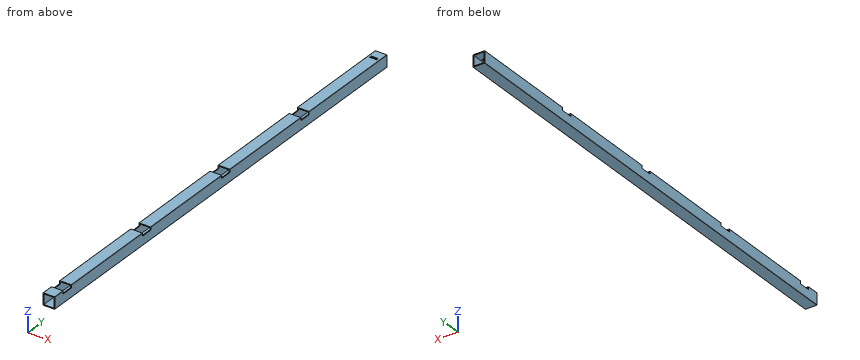
from build123d import *

# Parameters (mm, degrees)
SKETCH1_W           = 17
SKETCH1_H           = 17
BOSS_EXTRUDE1_DEPTH = 796.5
SKETCH3_W           = 12
SKETCH3_H           = 4
CUT_EXTRUDE1_DEPTH  = 10
SKETCH5_W           = 5
SKETCH5_H           = 20
CUT_EXTRUDE2_DEPTH  = 798.002038893


with BuildPart() as part:
    # Sketch1 → Boss-Extrude1 (new body)
    with BuildSketch(Plane(origin=(0, 0, 0), x_dir=(1, 0, 0), z_dir=(0, 1, 0))):
        with BuildLine():
            Line((0.5, 0), (19.5, 0))
            ThreePointArc((19.5, 0), (19.853553391, 0.146446609), (20, 0.5))
            Line((20, 0.5), (20, 19.5))
            ThreePointArc((20, 19.5), (19.853553391, 19.853553391), (19.5, 20))
            Line((19.5, 20), (0.5, 20))
            ThreePointArc((0.5, 20), (0.146446609, 19.853553391), (0, 19.5))
            Line((0, 19.5), (0, 0.5))
            ThreePointArc((0, 0.5), (0.146446609, 0.146446609), (0.5, 0))
        make_face()
        with Locations((10, 10)):
            Rectangle(SKETCH1_W, SKETCH1_H, mode=Mode.SUBTRACT)
    extrude(amount=BOSS_EXTRUDE1_DEPTH)

    # Sketch3 → Cut-Extrude1 (cut)
    with BuildSketch(Plane.XY):
        with Locations((10, 779.5)):
            Rectangle(SKETCH3_W, SKETCH3_H)
    extrude(amount=-CUT_EXTRUDE1_DEPTH, mode=Mode.SUBTRACT)

    # Sketch5 → Cut-Extrude2 (cut, through all)
    with BuildSketch(Plane.ZY):
        with Locations((-2.5, 600)):
            Rectangle(SKETCH5_W, SKETCH5_H)
        with Locations((-2.5, 410)):
            Rectangle(SKETCH5_W, SKETCH5_H)
        with Locations((-2.5, 220)):
            Rectangle(SKETCH5_W, SKETCH5_H)
        with Locations((-2.5, 30)):
            Rectangle(SKETCH5_W, SKETCH5_H)
    extrude(amount=-CUT_EXTRUDE2_DEPTH, mode=Mode.SUBTRACT)


solid = part.part
Design review of the part built by this model. Coordinates are the model's own, in mm. Round coordinates to 2 decimals unless told otherwise and drop trailing zeros. Write each loop counter-clockwise with the first axis right and the second up, starting at its lowest first coordinate (ties: lowest second). Pieces come first, ordered by that corner, then holes. Notation, with made-up numbers: (28.5, -6) - (80.5, -6) arc R24 ccw to (80.5, 24) - close; hole circle Ø6 at (56.5, 23.5). An arc over 180 degrees is marked (long way). Return JSON: item names as keys, results as strings. Group by question number.
Item 1: We need section B-B on z = -13.25. Write out the cut boundary in (x, y).
Item 2: Insertion check: P1, Ø0.8, axis at x = 19.5, y = 600, coming from the +Z side; P2, Ø6, axis at x = 7.5, z = -13, coming from the +Y side; P3, Ø5.5, axis at x = 5, z = -3, coming from the +Y side. Each pin has a flat end and moves straight along its axis. Give the tip position at first contact, or say it passes through.
Item 3: For probe 1 along Y at (x, z) = (1, -4); probe 2 along Z at (x, y) = (17, 636); probe 3 along X at (y, z) = (57.5, -17.5), list the stretches that pass through material, from the lowest coordinate up. Write a range as [from, to].
Item 4: We need section A-A on y = 715.5. Write out the cut boundary in (x, z), and give its area (3 significant figures).
Model answer:
{
 "1": {"outline": "(0, 0) - (1.5, 0) - (1.5, 796.5) - (0, 796.5) - close; (18.5, 0) - (20, 0) - (20, 796.5) - (18.5, 796.5) - close"},
 "2": {"P1": "stops at z = -5", "P2": "passes through", "P3": "stops at y = 796.5"},
 "3": {"probe 1": "y = [0, 20], [40, 210], [230, 400], [420, 590], [610, 796.5]", "probe 2": "z = [-20, -18.5], [-1.5, 0]", "probe 3": "x = [0, 1.5], [18.5, 20]"},
 "4": {"outline": "(0, -19.5) arc R0.5 ccw to (0.5, -20) - (19.5, -20) arc R0.5 ccw to (20, -19.5) - (20, -0.5) arc R0.5 ccw to (19.5, 0) - (0.5, 0) arc R0.5 ccw to (0, -0.5) - close; hole (1.5, -18.5) - (18.5, -18.5) - (18.5, -1.5) - (1.5, -1.5) - close", "area": "111 mm²"}
}
